Drawing for the job (mm, zero at the part's lowest x, y, z). A direction names the side the tool comes from. Coordinates: 2 decimals unless noted, no trailing zeros. Loops run counter-clockwise (first coordinate to the right, second up) from the corner with the lowest first, then second, coordinate; pieces in that order, holes last. Notation, with made-up numbers: (-20.75, 40) - (1.25, 40) arc R15 ccw to (1.25, 63) - close; hole circle Ø9 at (41.5, -22). An arc over 180 degrees is marked (long way). Put each result on its own line as item: value.
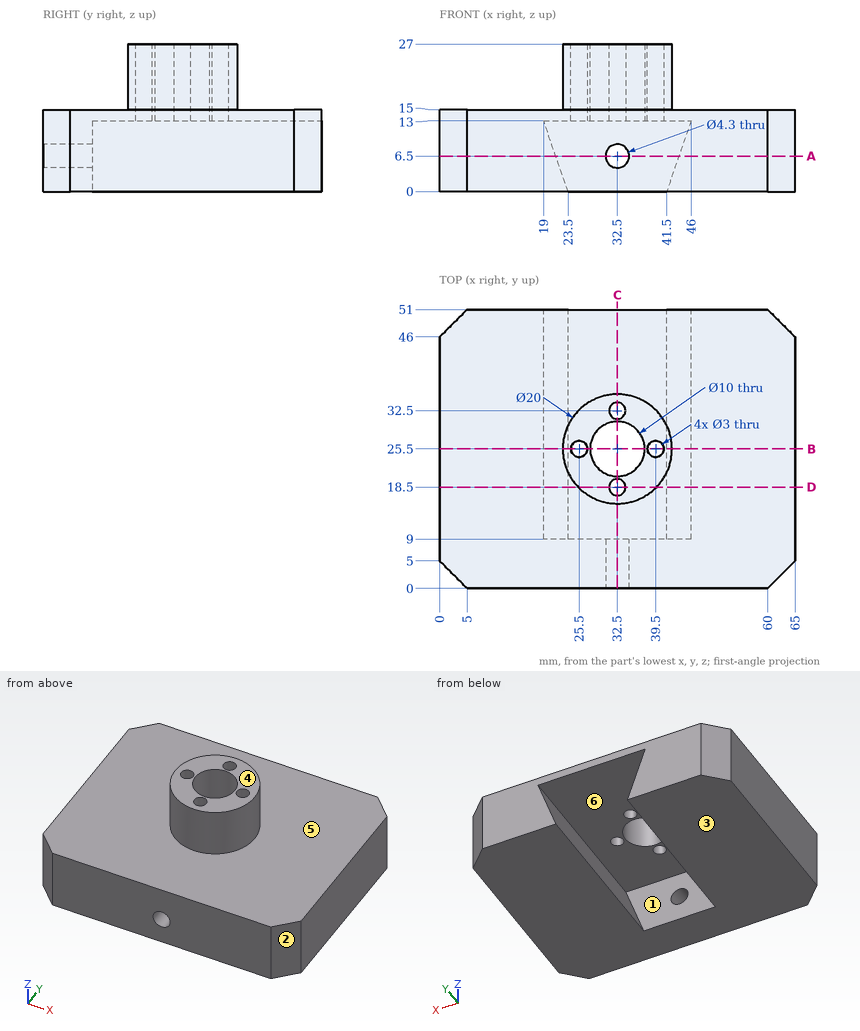
Q1. Wall check: L1, parallel to Y at x = 32.5, z = 19.25; L2, parallel to Z at x = 14.5, y = 26.5; L3, parallel to Z at x = 29.5, y = 36.5. Give the ranges that are in metal, low to high. Write a range as from..to.
Determined:
L1: 15.5..17, 20..20.5, 30.5..31, 34..35.5
L2: 0..15
L3: 13..15
Q2. Pin check, flat tips, straight feed: pin 1 Ø1.5 at (y, z) = (24, 21.5) entering from -X; pin 2 Ø4 at (x, y) = (36, 35.5) entering from -Z; pin 3 Ø5 at (x, y) = (19.5, 26.5) entering from +Z. Stop position of each tip, or through.
Determined:
pin 1: x = 22.53
pin 2: z = 13
pin 3: z = 15
Q3. Tool access for the marked faces 4, 5 and 6: list every direction of +Z, -Z, +X, -X, +Y, -Y with a clear straight run to the whole face (end or side of a thin tool).
Determined:
face 4: +Z, +X, -X, +Y, -Y
face 5: +Z
face 6: +Y
Q4. Mould opens along X. For the marked faces 1, 2 and 3 say: +X half, -X half, draft (parallel to the pull), parting line (faces both ways), or undercut.
Determined:
face 1: undercut
face 2: +X half
face 3: draft
Q5. Slice it at B-B, the plane y = 25.5. Give the cut face in (x, z).
Determined:
outline: (0, 0) - (23.5, 0) - (19, 13) - (24, 13) - (24, 27) - (22.5, 27) - (22.5, 15) - (0, 15) - close; (27, 13) - (27.5, 13) - (27.5, 27) - (27, 27) - close; (37.5, 13) - (38, 13) - (38, 27) - (37.5, 27) - close; (41, 13) - (46, 13) - (41.5, 0) - (65, 0) - (65, 15) - (42.5, 15) - (42.5, 27) - (41, 27) - close
Q6. Slice it at C-C, the plane x = 32.5. Give the cut face in (y, z).
Determined:
outline: (0, 0) - (9, 0) - (9, 4.35) - (0, 4.35) - close; (0, 8.65) - (9, 8.65) - (9, 13) - (17, 13) - (17, 27) - (15.5, 27) - (15.5, 15) - (0, 15) - close; (20, 13) - (20.5, 13) - (20.5, 27) - (20, 27) - close; (30.5, 13) - (31, 13) - (31, 27) - (30.5, 27) - close; (34, 13) - (51, 13) - (51, 15) - (35.5, 15) - (35.5, 27) - (34, 27) - close
Q7. Slice it at D-D, the plane y = 18.5. Give the cut face in (x, z).
Determined:
outline: (0, 0) - (23.5, 0) - (19, 13) - (31, 13) - (31, 27) - (25.36, 27) - (25.36, 15) - (0, 15) - close; (34, 13) - (46, 13) - (41.5, 0) - (65, 0) - (65, 15) - (39.64, 15) - (39.64, 27) - (34, 27) - close
Q8. Slice it at A-A, the plane z = 6.5. Give the cut face in (x, y).
Determined:
outline: (0, 5) - (5, 0) - (30.35, 0) - (30.35, 9) - (21.25, 9) - (21.25, 51) - (5, 51) - (0, 46) - close; (34.65, 0) - (60, 0) - (65, 5) - (65, 46) - (60, 51) - (43.75, 51) - (43.75, 9) - (34.65, 9) - close
